Read the model definition and answer for the solid it produces. Units are mm, in the model's axes. Round coordinates to 2 decimals unless told otherwise and drop trailing zeros. Order: outer loops, then holes, each group sorted by start corner. A loop starts at its lowest first (then second) coordinate and runs counter-clockwise, first axis right, second up. Notation, with made-up numbers: (22.5, -3) -> (71.5, -3) arc R14 ccw to (71.5, 12) -> close; hole circle Ø7 at (-18, 5.25). An arc over 180 degrees is marked (long way). Answer as a JSON object with one key per item and string values. Group by question number.
Item 1: Consider probe 1 along X at (y, z) = (14.5, -275); probe 2 along Z at (x, y) = (158, 18); probe 3 along Z at (x, y) = (16, 15.75). Determine where each line is inside the solid, lowest interval first. Write a range as from..to.
Item 2: Given P1, Ø23, axis at x = 25, z = -25, coming from the +Y side, flat-ended and moving along its own axis, determine where the tip first touches the part or whether it passes through.
Item 3: Section A-A, the plane x = 25 is taken. Write down the section's boundary in (y, z), plus the area to 3 significant figures.
Item 4: Section D-D, the plane z = -279.5 is taken. Count the separate pieces of the cut face and the enclosed holes in it, plus the area to 3 significant figures.
Item 5: The mould has two halves that part along Z. Classify faces 1 (the cylindrical face through (28, 11.66, -15.46)), 2 (the flat face through (89, 12, 0)), 3 (the conical face through (3.87, 0.57, -295.99)): pulls with the +Z half, pulls with the -Z half, needs draft (parallel to the pull), parting line crosses it, or undercut.
Item 6: Section B-B, the plane z = -25 is taken. Write down the section's boundary in (x, y), plus the area to 3 significant figures.
Item 7: Section C-C, the plane y = 10 is taken. Write down the section's boundary in (x, z).
from build123d import *

# Parameters (mm, degrees)
SKETCH1_W           = 180
SKETCH1_H           = 300
BOSS_EXTRUDE1_DEPTH = 25
SKETCH2_R           = 10
CUT_EXTRUDE1_DEPTH  = 351.749198146
FILLET1_R           = 10
CHAMFER2_SIZE       = 2
CHAMFER3_SIZE       = 2


with BuildPart() as part:
    # Sketch1 → Boss-Extrude1 (new body)
    with BuildSketch(Plane(origin=(0, 0, 0), x_dir=(1, 0, 0), z_dir=(0, 1, 0))):
        with Locations((90, 150)):
            Rectangle(SKETCH1_W, SKETCH1_H)
    extrude(amount=BOSS_EXTRUDE1_DEPTH)

    # Sketch2 → Cut-Extrude1 (cut, through all)
    with BuildSketch(Plane(origin=(0, 25, 0), x_dir=(1, 0, 0), z_dir=(0, 1, 0))):
        with Locations(Location((25, 25, 0), (0, 0, 270))):
            Circle(SKETCH2_R)
        with Locations(Location((155, 25, 0), (0, 0, 270))):
            Circle(SKETCH2_R)
        with Locations(Location((155, 150, 0), (0, 0, 270))):
            Circle(SKETCH2_R)
        with Locations(Location((155, 275, 0), (0, 0, 270))):
            Circle(SKETCH2_R)
        with Locations(Location((25, 150, 0), (0, 0, 270))):
            Circle(SKETCH2_R)
        with Locations(Location((25, 275, 0), (0, 0, 270))):
            Circle(SKETCH2_R)
    extrude(amount=-CUT_EXTRUDE1_DEPTH, mode=Mode.SUBTRACT)

    # Fillet1
    fillet1_edges = [part.edges().sort_by_distance(p)[0] for p in [
        (0, 12.5, -300),
        (180, 12.5, -300),
        (180, 12.5, 0),
        (0, 12.5, 0),
    ]]
    fillet(fillet1_edges, radius=FILLET1_R)

    # Chamfer2
    chamfer2_edges = [part.edges().sort_by_distance(p)[0] for p in [
        (90, 0, -300),
        (90, 25, -300),
        (0, 0, -150),
        (180, 0, -150),
        (90, 0, 0),
        (177.071067812, 0, -2.928932188),
        (2.928932188, 0, -2.928932188),
        (2.928932188, 0, -297.071067812),
        (177.071067812, 0, -297.071067812),
        (180, 25, -150),
        (0, 25, -150),
        (90, 25, 0),
        (177.071067812, 25, -2.928932188),
        (2.928932188, 25, -2.928932188),
        (2.928932188, 25, -297.071067812),
        (177.071067812, 25, -297.071067812),
    ]]
    chamfer(chamfer2_edges, length=CHAMFER2_SIZE)

    # Chamfer3
    chamfer3_edges = [part.edges().sort_by_distance(p)[0] for p in [
        (25, 25, -160),
        (155, 25, -285),
        (155, 25, -160),
        (155, 25, -35),
        (25, 25, -285),
        (25, 25, -35),
    ]]
    chamfer(chamfer3_edges, length=CHAMFER3_SIZE)


solid = part.part
Values found:
{
 "1": {"probe 1": "0..15, 35..145, 165..180", "probe 2": "-300..-284.54, -265.46..-159.54, -140.46..-34.54, -15.46..0", "probe 3": "-300..-279.36, -270.64..-154.36, -145.64..-29.36, -20.64..0"},
 "2": {"P1": "y = 24.5"},
 "3": {"outline": "(0, -298) -> (2, -300) -> (23, -300) -> (25, -298) -> (25, -287) -> (23, -285) -> (0, -285) -> close; (0, -265) -> (23, -265) -> (25, -263) -> (25, -162) -> (23, -160) -> (0, -160) -> close; (0, -140) -> (23, -140) -> (25, -138) -> (25, -37) -> (23, -35) -> (0, -35) -> close; (0, -15) -> (23, -15) -> (25, -13) -> (25, -2) -> (23, 0) -> (2, 0) -> (0, -2) -> close", "area": "5,980 mm2"},
 "4": {"separate pieces": "3", "enclosed holes": "0", "area": "3,590 mm2"},
 "5": {"face 1": "undercut", "face 2": "pulls with the +Z half", "face 3": "pulls with the -Z half"},
 "6": {"outline": "(0, 2) -> (2, 0) -> (15, 0) -> (15, 23) -> (13, 25) -> (2, 25) -> (0, 23) -> close; (35, 0) -> (145, 0) -> (145, 23) -> (143, 25) -> (37, 25) -> (35, 23) -> close; (165, 0) -> (178, 0) -> (180, 2) -> (180, 23) -> (178, 25) -> (167, 25) -> (165, 23) -> close", "area": "3,480 mm2"},
 "7": {"outline": "(0, -290) arc R10 ccw to (10, -300) -> (170, -300) arc R10 ccw to (180, -290) -> (180, -10) arc R10 ccw to (170, 0) -> (10, 0) arc R10 ccw to (0, -10) -> close; hole circle Ø20 at (25, -275); hole circle Ø20 at (25, -150); hole circle Ø20 at (25, -25); hole circle Ø20 at (155, -275); hole circle Ø20 at (155, -150); hole circle Ø20 at (155, -25)"}
}
